from build123d import *

# Parameters (mm, degrees)
SKETCH8_R                       = 4.5
BOSS_EXTRUDE2_DEPTH             = 7
SKETCH10_R                      = 6.55
CUT_EXTRUDE6_DEPTH              = 5
CUT_EXTRUDE7_DEPTH              = 10
CUT_EXTRUDE7_DEPTH_BACK         = 10
SKETCH11_R                      = 1.9
BOSS_EXTRUDE3_REACH             = 62.716
SKETCH12_R                      = 1.9
BOSS_EXTRUDE3_DIRECTION_2_REACH = 62.716
CUT_EXTRUDE8_REACH              = 65.597


with BuildPart() as part:
    # Sketch8 → Boss-Extrude2 (new body)
    with BuildSketch(Plane(origin=(0, 0, 0), x_dir=(1, 0, 0), z_dir=(0, 1, 0))):
        with BuildLine():
            Line((40, -5.5), (48.935186127, -9.490451592))
            ThreePointArc((48.935186127, -9.490451592), (59.55, 0), (48.935186127, 9.490451592))
            Line((48.935186127, 9.490451592), (40, 5.5))
            Line((40, 5.5), (0, 4))
            Line((0, 4), (0, -4))
            Line((0, -4), (40, -5.5))
        make_face()
        with Locations(Location((50, 0, 0), (0, 0, 270))):
            Circle(SKETCH8_R, mode=Mode.SUBTRACT)
    extrude(amount=BOSS_EXTRUDE2_DEPTH)

    # Sketch10 → Cut-Extrude6 (cut)
    with BuildSketch(Plane(origin=(0, 7, 0), x_dir=(1, 0, 0), z_dir=(0, 1, 0))):
        with Locations(Location((50, 0, 0), (0, 0, 270))):
            Circle(SKETCH10_R)
    extrude(amount=-CUT_EXTRUDE6_DEPTH, mode=Mode.SUBTRACT)

    # Sketch11 → Cut-Extrude7 (cut, two sides: drawn at the far end of the back side and taken through both)
    with BuildSketch(Plane.XY.offset(-CUT_EXTRUDE7_DEPTH_BACK)):
        with Locations(Location((5, 4, 0), (0, 0, 180))):
            Circle(SKETCH11_R)
        with Locations(Location((15, 4, 0), (0, 0, 180))):
            Circle(SKETCH11_R)
    extrude(amount=CUT_EXTRUDE7_DEPTH + CUT_EXTRUDE7_DEPTH_BACK, mode=Mode.SUBTRACT)

    # Boss-Extrude3: up to this plane
    boss_extrude3_end = Plane(origin=(-0.149789359, 7, 3.994382899), z_dir=(0.037473660589094265, 0, -0.9992976157091807))
    # Sketch12 → Boss-Extrude3 (add, up to the surface)
    with BuildSketch(Plane.XY, mode=Mode.PRIVATE) as boss_extrude3_sk1:
        Polygon((23.894935943, 7), (13.540419669, 20.177956538), (0, 20.177956538), (0, 7), align=None)
        with Locations(Location((8.136364364, 16.418485591, 0), (0, 0, 180))):
            Circle(SKETCH12_R, mode=Mode.SUBTRACT)
    boss_extrude3_tool1 = split(extrude(boss_extrude3_sk1.sketch, amount=BOSS_EXTRUDE3_REACH, mode=Mode.PRIVATE), bisect_by=boss_extrude3_end, keep=Keep.BOTH, mode=Mode.PRIVATE)
    add(boss_extrude3_tool1.solids().sort_by_distance((9.667927, 12.815835, 0))[0])

    # Boss-Extrude3 direction 2: up to this plane
    boss_extrude3_direction_2_end = Plane(origin=(-0.149789359, 7, -3.994382899), z_dir=(-0.037473660589094265, 0, -0.9992976157091807))
    # Sketch12 → Boss-Extrude3 direction 2 (add, up to the surface)
    with BuildSketch(Plane.XY, mode=Mode.PRIVATE) as boss_extrude3_direction_2_sk1:
        Polygon((23.894935943, 7), (13.540419669, 20.177956538), (0, 20.177956538), (0, 7), align=None)
        with Locations(Location((8.136364364, 16.418485591, 0), (0, 0, 180))):
            Circle(SKETCH12_R, mode=Mode.SUBTRACT)
    boss_extrude3_direction_2_tool1 = split(extrude(boss_extrude3_direction_2_sk1.sketch, amount=-BOSS_EXTRUDE3_DIRECTION_2_REACH, mode=Mode.PRIVATE), bisect_by=boss_extrude3_direction_2_end, keep=Keep.BOTH, mode=Mode.PRIVATE)
    add(boss_extrude3_direction_2_tool1.solids().sort_by_distance((9.667927, 12.815835, 0))[0])

    # Cut-Extrude8: up to this face of the body (flat: up to its plane)
    cut_extrude8_end = Plane(part.part.faces().sort_by_distance((6.904897785, 20.177956538, 0))[0])
    # Sketch13 → Cut-Extrude8 (cut, up to the picked face)
    with BuildSketch(Plane(origin=(0, 0, 0), x_dir=(1, 0, 0), z_dir=(0, 1, 0)), mode=Mode.PRIVATE) as cut_extrude8_sk1:
        Polygon((8.018762989, 0), (37.792949753, 2.126727626), (37.792949753, -2.126727626), align=None)
    cut_extrude8_tool1 = split(extrude(cut_extrude8_sk1.sketch, amount=CUT_EXTRUDE8_REACH, mode=Mode.PRIVATE), bisect_by=cut_extrude8_end, keep=Keep.BOTH, mode=Mode.PRIVATE)
    add(cut_extrude8_tool1.solids().sort_by(Axis((27.868221, 0, 0), (0, 1, 0)))[0], mode=Mode.SUBTRACT)


solid = part.part
Geometry: final body of the model. Coordinates: model frame, mm. A direction names the side the tool comes from. Give positions to 0.01 mm unless a question says otherwise; leave off trailing zeros. Loops run counter-clockwise (first coordinate to the right, second up) from the corner with the lowest first, then second, coordinate; pieces in that order, holes last. Notation, with made-up numbers: (44.5, 78) -> (90.5, 78) arc R12 cw to (90.5, 96) -> close; hole circle Ø7 at (12.5, -26). An arc over 180 degrees is marked (long way). Put each result on its own line as item: value.
1. Pull-direction query (X, two-part tool) for faces 1 (the flat face through (41, 7, 0)), 2 (the cylindrical face through (6.324, 15.848, 0.061)), 3 (the flat face through (0, 10, 0)); classes: released by +X, released by -X, zero draft, split by the parting line, or undercut.
Taken from the geometry:
face 1: zero draft
face 2: undercut
face 3: released by -X
2. Cut plane C-C (x = 50). Return the cut outline in (y, z).
Taken from the geometry:
outline: (0, -9.55) -> (7, -9.55) -> (7, -6.55) -> (2, -6.55) -> (2, -4.5) -> (0, -4.5) -> close; (0, 4.5) -> (2, 4.5) -> (2, 6.55) -> (7, 6.55) -> (7, 9.55) -> (0, 9.55) -> close
3. Pin query (flat end, axial travel): P1, Ø5, axis at x = 36.5, y = 9, coming from the -Z side (3 decimals); P2, Ø4, axis at x = 48.5, z = 2.5, coming from the +Y side; P3, Ø5, axis at x = 5, y = 4, coming from the -Z side; P4, Ø1, axis at y = 17, z = -6, coming from the +X side. Return the tip coordinate at first contact, or that it passes through.
Taken from the geometry:
P1: stops at z = -5.425
P2: stops at y = 2
P3: stops at z = -4.28
P4: passes through
4. Cut plane D-D (x = 28.5). Return the cut outline in (y, z), plus the area to 3 significant figures.
Taken from the geometry:
outline: (0, -5.07) -> (7, -5.07) -> (7, -1.46) -> (0, -1.46) -> close; (0, 1.46) -> (7, 1.46) -> (7, 5.07) -> (0, 5.07) -> close
area: 50.5 mm2
5. Cut plane A-A (z = 2.75). Return the cut outline in (x, y), plus the area to 3 significant figures.
Taken from the geometry:
outline: (0, 0) -> (46.44, 0) -> (46.44, 2) -> (44.06, 2) -> (44.06, 7) -> (23.89, 7) -> (13.54, 20.18) -> (0, 20.18) -> close; (53.56, 0) -> (59.15, 0) -> (59.15, 7) -> (55.94, 7) -> (55.94, 2) -> (53.56, 2) -> close; hole circle Ø3.8 at (5, 4); hole circle Ø3.8 at (8.14, 16.42); hole circle Ø3.8 at (15, 4)
area: 553 mm2
6. Ray query, line 1 along X through (y, z) = (4, -3.45); line 2 along Y through (x, z) = (15, -2.95); line 3 along Z through (x, y) = (13.5, 10.25). Return the intervals inside material, ascending. Write a range as [from, to].
Taken from the geometry:
line 1: x = [0, 3.1], [6.9, 13.1], [16.9, 44.43], [55.57, 58.91]
line 2: y = [0, 2.1], [5.9, 18.32]
line 3: z = [-4.51, -0.39], [0.39, 4.51]
7. Set-up query: faces 4 (the flat face through (37.793, 3, 0)), 5 (the flat face through (36, 0, -2.3)), 6 (the cylindrical face through (43.6, 4.5, -1.4)). Return all of +Z, -Z, +X, -X, +Y, -Y with unobstructed straight access to the full face (end or side cutting, diameter ignored); none if empty.
Taken from the geometry:
face 4: +Y, -Y
face 5: +Z, -Z, +X, -X, -Y
face 6: +Y
8. Cut plane B-B (y = 4). Return the cut outline in (x, z).
Taken from the geometry:
outline: (0, -4) -> (3.1, -4.12) -> (3.1, 4.12) -> (0, 4) -> close; (6.9, -4.26) -> (13.1, -4.49) -> (13.1, -0.36) -> (8.02, 0) -> (13.1, 0.36) -> (13.1, 4.49) -> (6.9, 4.26) -> close; (16.9, -4.63) -> (40, -5.5) -> (48.94, -9.49) arc R9.55 ccw (long way) to (48.94, 9.49) -> (40, 5.5) -> (16.9, 4.63) -> (16.9, 0.63) -> (37.79, 2.13) -> (37.79, -2.13) -> (16.9, -0.63) -> close; hole circle Ø13.1 at (50, 0)
